Geometry check sheet. Reference: drawing and pictorial views, mm from the part's lowest x, y, z. A direction names the side the tool comes from. Coordinates: 2 decimals unless noted, no trailing zeros. Write each loop counter-clockwise with the first axis right and the second up, starting at its lowest first coordinate (ties: lowest second). Pieces come first, ordered by that corner, then holes. Notation, with made-up numbers: (64, 59) - (117, 59) arc R26 ccw to (117, 92) - close; hole circle Ø1 at (80, 32.25). An arc over 180 degrees is marked (long way). Use one line per item in the form item = value. Start each with the question number.
(1) Sectioned sample at C-C (y = 36.5). Record the cut outline in (x, z) (3 decimals).
(2) Sectioned sample at D-D (x = 35.5). Record the cut outline in (y, z) (3 decimals), and give its area (3 significant figures).
(3) Gauge pin test, flat ends, axial feed: pin 1 Ø6.5 at (y, z) = (15, 6.5) entering from +X; pin 2 Ø4 at (y, z) = (23, 4) entering from -X (3 decimals); pin 3 Ø5.5 at (x, z) = (10, 6.35) entering from +Y. Record the tip position at first contact, or that the pin passes through.
(4) Material ranges on line 1 (Z direction, x = 10, y = 2.2); line 2 (X direction, y = 28.5, z = 4) (3 decimals); line 3 (Y direction, x = 88.5, z = 5.5) (3 decimals), recorded low to high. Write a range as [from, to].
(5) Sectioned sample at A-A (x = 10). Record the cut outline in (y, z) (3 decimals), and give its area (3 significant figures).
(6) Tool access check on the marked faces 1, 2 and 3. Record the directions out of +Z, -Z, +X, -X, +Y, -Y that give a thin tool (end or side, any length) a straight path to the whole face; none if there is none.
(7) Sectioned sample at B-B (z = 6.35). Record the cut outline in (x, y) (3 decimals), and give its area (3 significant figures).
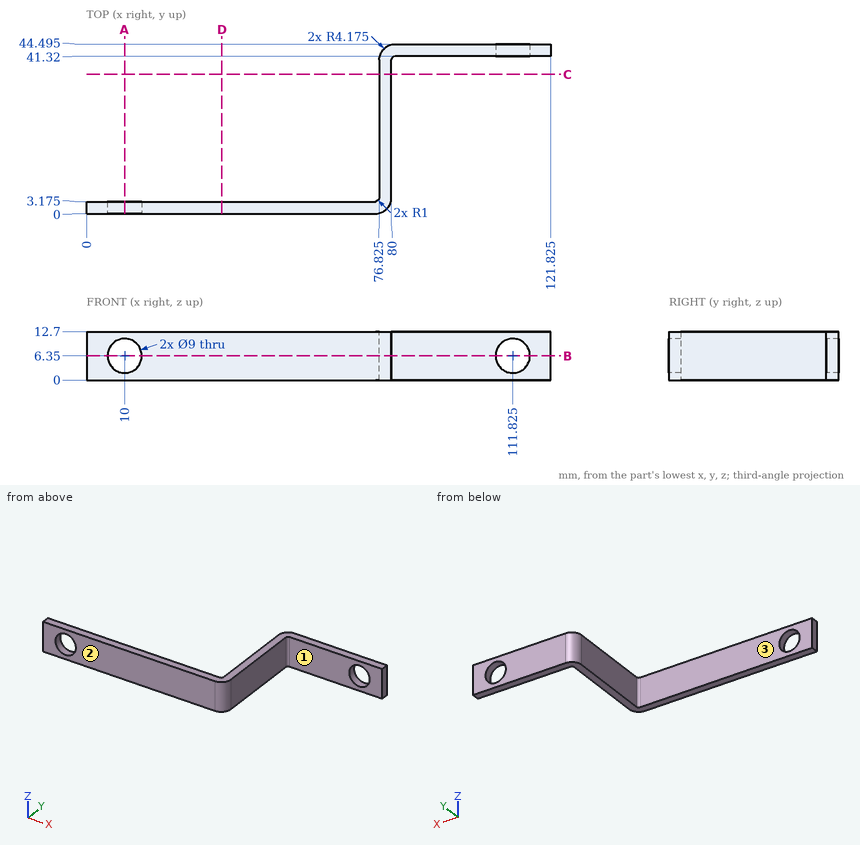
Answers below:
q1.outline = (76.825, 0) - (80, 0) - (80, 12.7) - (76.825, 12.7) - close
q2.outline = (0, 0) - (3.175, 0) - (3.175, 12.7) - (0, 12.7) - close
q2.area = 40.3 mm2
q3.pin_1 = 80
q3.pin_2 = 76.825
q3.pin_3 = through
q4.line_1 = [0, 1.85], [10.85, 12.7]
q4.line_2 = [76.825, 80]
q4.line_3 = [41.32, 44.495]
q5.outline = (0, 0) - (3.175, 0) - (3.175, 1.85) - (0, 1.85) - close; (0, 10.85) - (3.175, 10.85) - (3.175, 12.7) - (0, 12.7) - close
q5.area = 11.7 mm2
q6.face_1 = +Z, -Z, +X, -Y
q6.face_2 = +Z, -Z, +X, -X, -Y
q6.face_3 = +Z, -Z, -X, +Y
q7.outline = (0, 0) - (5.5, 0) - (5.5, 3.175) - (0, 3.175) - close; (14.5, 0) - (75.825, 0) arc R4.175 ccw to (80, 4.175) - (80, 40.32) arc R1 cw to (81, 41.32) - (107.325, 41.32) - (107.325, 44.495) - (81, 44.495) arc R4.175 ccw to (76.825, 40.32) - (76.825, 4.175) arc R1 cw to (75.825, 3.175) - (14.5, 3.175) - close; (116.325, 41.32) - (121.825, 41.32) - (121.825, 44.495) - (116.325, 44.495) - close
q7.area = 454 mm2
